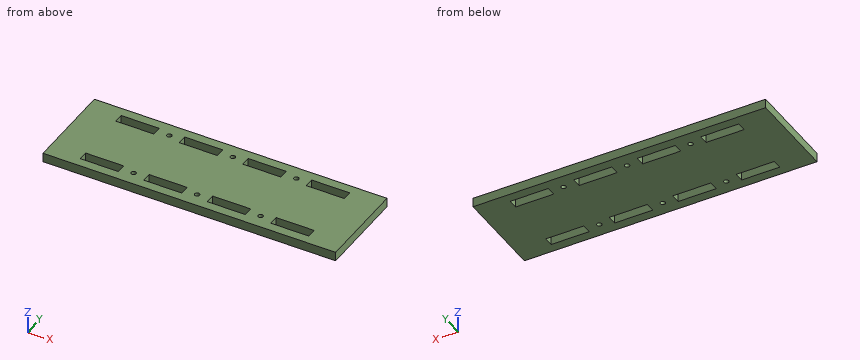
```python
from build123d import *

# Parameters (mm, degrees)
SKETCH1_W           = 192
SKETCH1_H           = 59.4
SKETCH1_R           = 1.6
SKETCH1_W_2         = 25
SKETCH1_H_2         = 6.2
BOSS_EXTRUDE1_DEPTH = 6


with BuildPart() as part:
    # Sketch1 → Boss-Extrude1 (new body)
    with BuildSketch(Plane.XY):
        Rectangle(SKETCH1_W, SKETCH1_H)
        with Locations((-41.666666667, -20.6)):
            Circle(SKETCH1_R, mode=Mode.SUBTRACT)
        with Locations((0, -20.6)):
            Circle(SKETCH1_R, mode=Mode.SUBTRACT)
        with Locations((41.666666667, -20.6)):
            Circle(SKETCH1_R, mode=Mode.SUBTRACT)
        with Locations((0, 20.6)):
            Circle(SKETCH1_R, mode=Mode.SUBTRACT)
        with Locations((41.666666667, 20.6)):
            Circle(SKETCH1_R, mode=Mode.SUBTRACT)
        with Locations((-41.666666667, 20.6)):
            Circle(SKETCH1_R, mode=Mode.SUBTRACT)
        with Locations((-20.833333333, -20.6)):
            Rectangle(SKETCH1_W_2, SKETCH1_H_2, mode=Mode.SUBTRACT)
        with Locations((-62.5, -20.6)):
            Rectangle(SKETCH1_W_2, SKETCH1_H_2, mode=Mode.SUBTRACT)
        with Locations((20.833333333, -20.6)):
            Rectangle(SKETCH1_W_2, SKETCH1_H_2, mode=Mode.SUBTRACT)
        with Locations((62.5, -20.6)):
            Rectangle(SKETCH1_W_2, SKETCH1_H_2, mode=Mode.SUBTRACT)
        with Locations((-62.5, 20.6)):
            Rectangle(SKETCH1_W_2, SKETCH1_H_2, mode=Mode.SUBTRACT)
        with Locations((-20.833333333, 20.6)):
            Rectangle(SKETCH1_W_2, SKETCH1_H_2, mode=Mode.SUBTRACT)
        with Locations((20.833333333, 20.6)):
            Rectangle(SKETCH1_W_2, SKETCH1_H_2, mode=Mode.SUBTRACT)
        with Locations((62.5, 20.6)):
            Rectangle(SKETCH1_W_2, SKETCH1_H_2, mode=Mode.SUBTRACT)
    extrude(amount=BOSS_EXTRUDE1_DEPTH)


solid = part.part
```
Read the model definition and answer for the solid it produces. Units are mm, in the model's axes. Give positions to 0.01 mm unless a question says otherwise; leave off trailing zeros. Order: outer loops, then holes, each group sorted by start corner. A loop starts at its lowest first (then second) coordinate and runs counter-clockwise, first axis right, second up. Notation, with made-up numbers: (75.5, -8) -> (101.5, -8) arc R15 ccw to (101.5, 4) -> close; hole circle Ø2 at (61, 50). An arc over 180 degrees is marked (long way). One line per item, written item: value. Start each with the question number.
(1) The part is cut by section A-A (x = -28.5). Determine the outline of the cut face in (y, z).
(2) A flat-ended cylindrical pin translates along its axis: P1, Ø2, axis at x = -28.5, y = 19.5, coming from the +Z side. Find the tip coordinate at first contact, or state that the pin passes through.
(3) Straight lines are drawn through the part: L1, parallel to Y at x = 59, z = 4.8; L2, parallel to Y at x = 0, z = 3.2; L3, parallel to X at y = 18.5, z = 0.95. For each, find the intervals that lie inside material, in ascending order.
Taken from the geometry:
1. outline: (-29.7, 0) -> (-23.7, 0) -> (-23.7, 6) -> (-29.7, 6) -> close; (-17.5, 0) -> (17.5, 0) -> (17.5, 6) -> (-17.5, 6) -> close; (23.7, 0) -> (29.7, 0) -> (29.7, 6) -> (23.7, 6) -> close
2. P1: through
3. L1: -29.7 to -23.7, -17.5 to 17.5, 23.7 to 29.7
3. L2: -29.7 to -22.2, -19 to 19, 22.2 to 29.7
3. L3: -96 to -75, -50 to -33.33, -8.33 to 8.33, 33.33 to 50, 75 to 96
